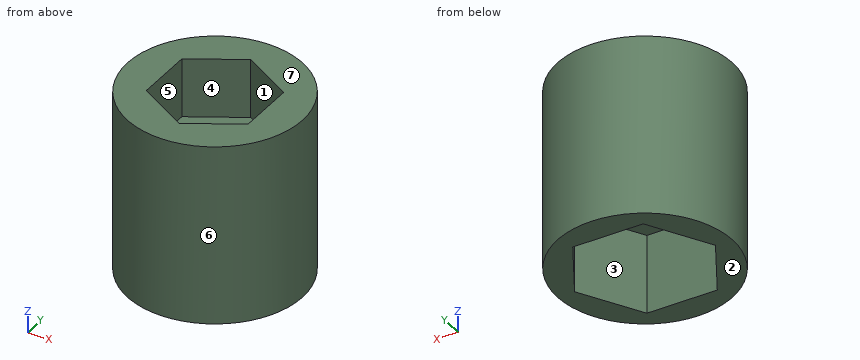
Autodesk Inventor part; units mm, degrees
ref_plane "Work Plane1" through (-12.7, 0, -12.7) normal (0, 0, 1) x (1, 0, 0)
ref_plane "Work Plane2" through (-11.7, 1, -12.7) normal (0, 0, 1) x (1, 0, 0)
ref_plane "Work Plane3" through (-8.125, -8.125, -9.7) normal (0, 0, 1) x (1, 0, 0)
sketch "Sketch2" plane through (0, 0, 0) normal (0, 0, 1) x (1, 0, 0)
  circle A0 centre (0, 0) radius 10.3923
  line L0 (-4.0415, -7) -> (4.0415, -7)
  line L1 (4.0415, -7) -> (8.0829, 0)
  line L2 (8.0829, 0) -> (4.0415, 7)
  line L3 (4.0415, 7) -> (-4.0415, 7)
  line L4 (-4.0415, 7) -> (-8.0829, 0)
  line L5 (-8.0829, 0) -> (-4.0415, -7)
  line L6 (4.0415, 7) -> (5.1962, 9) construction
  line L7 (-8.3716, 0) -> (-4.1858, -7.25)
  line L8 (-4.1858, -7.25) -> (4.1858, -7.25)
  line L9 (4.1858, -7.25) -> (8.3716, 0)
  line L10 (8.3716, 0) -> (4.1858, 7.25)
  line L11 (4.1858, 7.25) -> (-4.1858, 7.25)
  line L12 (-4.1858, 7.25) -> (-8.3716, 0)
  dimension "d9" = 2
  dimension "d10" = 0.25
  dimension "d11" = 0.25
  dimension "d12" = 0.25
  dimension "d13" = 0.25
  dimension "d14" = 0.25
  dimension "d15" = 0.25
ref_plane "Work Plane1" through (-12.7, 0, -12.7) normal (0, 0, 1) x (1, 0, 0)
ref_plane "Work Plane2" through (-11.7, 1, -12.7) normal (0, 0, 1) x (1, 0, 0)
ref_plane "Work Plane3" through (-8.125, -8.125, -9.7) normal (0, 0, 1) x (1, 0, 0)
extrude "Extrusion3" add sketch "Sketch2" against normal up to surface (9.7 mm away) contours A0
sketch "Sketch4" plane through (0, 0, 0) normal (0, 0, 1) x (1, 0, 0)
  circle A0 centre (0, 0) radius 10.3923
extrude "Extrusion4" add sketch "Sketch4" along normal blind 12
sketch "Sketch5" plane through (0, 0, -9.7) normal (0, 0, -1) x (-1, 0, 0)
  circle A0 centre (0, 0) radius 10.3923
  point P0 (0, 0)
extrude "Extrusion5" cut sketch "Sketch5" against normal blind 0.3
sketch "Sketch6" plane through (0, 0, 12) normal (0, 0, 1) x (1, 0, 0)
  line L0 (-6.05, 3.493) -> (0, 6.9859)
  line L1 (0, 6.9859) -> (6.05, 3.493)
  line L2 (6.05, 3.493) -> (6.05, -3.493)
  line L3 (6.05, -3.493) -> (0, -6.9859)
  line L4 (0, -6.9859) -> (-6.05, -3.493)
  line L5 (-6.05, -3.493) -> (-6.05, 3.493)
  line L6 (-14.5492, 0) -> (14.5492, 0)
  line L7 (0, -6.9859) -> (0, 6.9859) construction
  line L8 (6.05, -3.493) -> (-6.05, 3.493) construction
  line L9 (0, -14.5492) -> (0, 14.5492)
  point P0 (0, 0)
  point P1 (14.5492, 0)
  point P2 (0, 0)
  dimension "d32" = 0
  dimension "d35" = 12.1
extrude "Extrusion6" cut sketch "Sketch6" against normal blind 7
sketch "Sketch7" plane through (0, 0, 5) normal (0, 0, 1) x (1, 0, 0)
  circle A0 centre (0, 0) radius 2.15
  point P0 (0, 0)
  dimension "d21" = 4.3
extrude "Extrusion7" cut sketch "Sketch7" against normal through all
sketch "Sketch10" plane through (0, 0, 0) normal (0, 0, -1) x (-1, 0, 0)
  circle A0 centre (0, 0) radius 10.3923
  circle A1 centre (0, 0) radius 4.5
  dimension "d25" = 9
extrude "Extrusion8" cut sketch "Sketch10" against normal blind 1 contours A1
equation "\"d11\" = d10"
equation "\"d12\" = d11"
equation "\"d13\" = d12"
equation "\"d14\" = d13"
equation "\"d15\" = d14"
properties part number "ServoToScrewKey" material "ABS Plastic"
The model under review builds one solid part; all positions refer to its coordinate system, in mm. Face numbers are marked on the shaded views. A direction names the side the tool comes from. Round coordinates to 2 decimals unless told otherwise and drop trailing zeros. Order: outer loops, then holes, each group sorted by start corner. A loop starts at its lowest first (then second) coordinate and runs counter-clockwise, first axis right, second up. Notation, with made-up numbers: (0, -12) - (53, -12) arc R13 cw to (53, 12) - close; hole circle Ø8 at (72, -27). An arc over 180 degrees is marked (long way). Answer in a Markdown table with one row per item.
(1) Take a section at A-A on z = -6. Write out the cut boundary in (x, y), plus the area to 3 significant figures.
Result set:
| item | result |
|---|---|
| outline | circle Ø20.78 at (0, 0); hole (-8.37, 0) - (-4.19, -7.25) - (4.19, -7.25) - (8.37, 0) - (4.19, 7.25) - (-4.19, 7.25) - close |
| area | 157 mm2 |
(2) Take a section at D-D on y = -6. Write out the cut boundary in (x, z), plus the area to 3 significant figures.
Result set:
| item | result |
|---|---|
| outline | (-8.49, -9.4) - (-4.91, -9.4) - (-4.91, 0) - (4.91, 0) - (4.91, -9.4) - (8.49, -9.4) - (8.49, 12) - (1.71, 12) - (1.71, 5) - (-1.71, 5) - (-1.71, 12) - (-8.49, 12) - close |
| area | 247 mm2 |
(3) Take a section at B-B on y = -1. Write out the cut boundary in (x, z).
Result set:
| item | result |
|---|---|
| outline | (-10.34, -9.4) - (-7.79, -9.4) - (-7.79, 0) - (-4.39, 0) - (-4.39, 1) - (-1.9, 1) - (-1.9, 5) - (-6.05, 5) - (-6.05, 12) - (-10.34, 12) - close; (1.9, 1) - (4.39, 1) - (4.39, 0) - (7.79, 0) - (7.79, -9.4) - (10.34, -9.4) - (10.34, 12) - (6.05, 12) - (6.05, 5) - (1.9, 5) - close |
(4) Mouldability with a two-part tool opening along Y and no side actions: class the marked faces 4, 5, 6 and 7 as released by +Y, released by -Y, zero draft, split by the parting line, or undercut.
Result set:
| item | result |
|---|---|
| face 4 | undercut |
| face 5 | undercut |
| face 6 | split by the parting line |
| face 7 | zero draft |
(5) Take a section at C-C on x = 7.25. Write out the cut boundary in (y, z).
Result set:
| item | result |
|---|---|
| outline | (-7.45, -9.4) - (-1.94, -9.4) - (-1.94, 0) - (1.94, 0) - (1.94, -9.4) - (7.45, -9.4) - (7.45, 12) - (-7.45, 12) - close |
(6) Machinability: for the marked faces 1, 2 and 3, which of the approach directions +Z, -Z, +X, -X, +Y, -Y give a long, thin tool a straight path to every point of the face, cutting with its end or side? Answer none if there is none.
Result set:
| item | result |
|---|---|
| face 1 | +Z |
| face 2 | -Z, +X, -X, +Y, -Y |
| face 3 | -Z |
(7) For line 1 (Y direction, x = 0, z = 4); line 2 (Y direction, x = 0, z = 0.55); line 3 (X direction, y = 3.25, z = 10.75), list the stretches that pass through material, from the lowest coordinate up. Write a range as from..to.
Result set:
| item | result |
|---|---|
| line 1 | y = -10.39..-2.15, 2.15..10.39 |
| line 2 | y = -10.39..-4.5, 4.5..10.39 |
| line 3 | x = -9.87..-6.05, 6.05..9.87 |
(8) Clearance check with flat-ended pins moving along their axes: P1, Ø1, axis at y = -1, z = 0.5, coming from the -X side; P2, Ø7, axis at x = 0, y = 0, coming from the +Z side; P3, Ø1.5, axis at y = 3.5, z = 9, coming from the +X side. State where each tip first meets the part, or that it passes through.
Result set:
| item | result |
|---|---|
| P1 | stops at x = -10.38 |
| P2 | stops at z = 5 |
| P3 | stops at x = 10.02 |
